from build123d import *

# Parameters (mm, degrees)
F1_DEPTH       = 25
F3_DEPTH       = 5
F2_R           = 2
F4_DEPTH       = 7.001
F6_D           = 4
F6_CBORE_D     = 7.5
F6_CBORE_DEPTH = 2.5
F7_R           = 10
F8_DEPTH       = 2
F9_R           = 2.5


with BuildPart() as f1:
    # F0 (on Right) → F1 (new body)
    with BuildSketch(Plane.YZ):
        with BuildLine():
            Line((24, 25), (-24, 25))
            ThreePointArc((-24, 25), (-32.4852813742, 21.4852813742), (-36, 13))
            Line((-36, 13), (-36, 10))
            ThreePointArc((-36, 10), (-34.6554428129, 4.480802734), (-30.9230769231, 0.1984181931))
            ThreePointArc((-30.9230769231, 0.1984181931), (-30.6120464323, -0.1584471853), (-30.5, -0.6183802908))
            Line((-30.5, -0.6183802908), (-30.5, -41.5))
            ThreePointArc((-30.5, -41.5), (-30.2071067812, -42.2071067812), (-29.5, -42.5))
            Line((-29.5, -42.5), (-28.9142135624, -42.5))
            ThreePointArc((-28.9142135624, -42.5), (-28.53153013, -42.4238795325), (-28.2071067812, -42.2071067812))
            Line((-28.2071067812, -42.2071067812), (-26.2928932188, -40.2928932188))
            ThreePointArc((-26.2928932188, -40.2928932188), (-26.0761204675, -39.96846987), (-26, -39.5857864376))
            Line((-26, -39.5857864376), (-26, -39))
            Line((-26, -39), (-27, -39))
            Line((-27, -39), (-27, -37))
            Line((-27, -37), (-26, -37))
            Line((-26, -37), (-26, -36.4142135624))
            ThreePointArc((-26, -36.4142135624), (-26.0761204675, -36.03153013), (-26.2928932188, -35.7071067812))
            Line((-26.2928932188, -35.7071067812), (-28.2071067812, -33.7928932188))
            ThreePointArc((-28.2071067812, -33.7928932188), (-28.4238795325, -33.46846987), (-28.5, -33.0857864376))
            Line((-28.5, -33.0857864376), (-28.5, -11.4142135624))
            ThreePointArc((-28.5, -11.4142135624), (-28.4238795325, -11.03153013), (-28.2071067812, -10.7071067812))
            Line((-28.2071067812, -10.7071067812), (-27.7928932188, -10.2928932188))
            ThreePointArc((-27.7928932188, -10.2928932188), (-27.5761204675, -9.96846987), (-27.5, -9.5857864376))
            Line((-27.5, -9.5857864376), (-27.5, -9))
            Line((-27.5, -9), (-28.5, -9))
            Line((-28.5, -9), (-28.5, -7))
            Line((-28.5, -7), (-27.5, -7))
            Line((-27.5, -7), (-27.5, -6.4142135624))
            ThreePointArc((-27.5, -6.4142135624), (-27.5761204675, -6.03153013), (-27.7928932188, -5.7071067812))
            Line((-27.7928932188, -5.7071067812), (-28.2071067812, -5.2928932188))
            ThreePointArc((-28.2071067812, -5.2928932188), (-28.4238795325, -4.96846987), (-28.5, -4.5857864376))
            Line((-28.5, -4.5857864376), (-28.5, -2.5199840255))
            ThreePointArc((-28.5, -2.5199840255), (-28.1044705248, -1.7233565187), (-27.2307692308, -1.5569083313))
            ThreePointArc((-27.2307692308, -1.5569083313), (-25.6305060602, -1.8887110314), (-24, -2))
            Line((-24, -2), (24, -2))
            ThreePointArc((24, -2), (25.6305060602, -1.8887110314), (27.2307692308, -1.5569083313))
            ThreePointArc((27.2307692308, -1.5569083313), (28.1044705248, -1.7233565187), (28.5, -2.5199840255))
            Line((28.5, -2.5199840255), (28.5, -4.5857864376))
            ThreePointArc((28.5, -4.5857864376), (28.4238795325, -4.96846987), (28.2071067812, -5.2928932188))
            Line((28.2071067812, -5.2928932188), (27.7928932188, -5.7071067812))
            ThreePointArc((27.7928932188, -5.7071067812), (27.5761204675, -6.03153013), (27.5, -6.4142135624))
            Line((27.5, -6.4142135624), (27.5, -7))
            Line((27.5, -7), (28.5, -7))
            Line((28.5, -7), (28.5, -9))
            Line((28.5, -9), (27.5, -9))
            Line((27.5, -9), (27.5, -9.5857864376))
            ThreePointArc((27.5, -9.5857864376), (27.5761204675, -9.96846987), (27.7928932188, -10.2928932188))
            Line((27.7928932188, -10.2928932188), (28.2071067812, -10.7071067812))
            ThreePointArc((28.2071067812, -10.7071067812), (28.4238795325, -11.03153013), (28.5, -11.4142135624))
            Line((28.5, -11.4142135624), (28.5, -33.0857864376))
            ThreePointArc((28.5, -33.0857864376), (28.4238795325, -33.46846987), (28.2071067812, -33.7928932188))
            Line((28.2071067812, -33.7928932188), (26.2928932188, -35.7071067812))
            ThreePointArc((26.2928932188, -35.7071067812), (26.0761204675, -36.03153013), (26, -36.4142135624))
            Line((26, -36.4142135624), (26, -37))
            Line((26, -37), (27, -37))
            Line((27, -37), (27, -39))
            Line((27, -39), (26, -39))
            Line((26, -39), (26, -39.5857864376))
            ThreePointArc((26, -39.5857864376), (26.0761204675, -39.96846987), (26.2928932188, -40.2928932188))
            Line((26.2928932188, -40.2928932188), (28.2071067812, -42.2071067812))
            ThreePointArc((28.2071067812, -42.2071067812), (28.53153013, -42.4238795325), (28.9142135624, -42.5))
            Line((28.9142135624, -42.5), (29.5, -42.5))
            ThreePointArc((29.5, -42.5), (30.2071067812, -42.2071067812), (30.5, -41.5))
            Line((30.5, -41.5), (30.5, -0.6183802908))
            ThreePointArc((30.5, -0.6183802908), (30.6120464323, -0.1584471853), (30.9230769231, 0.1984181931))
            ThreePointArc((30.9230769231, 0.1984181931), (34.6554428129, 4.480802734), (36, 10))
            Line((36, 10), (36, 13))
            ThreePointArc((36, 13), (32.4852813742, 21.4852813742), (24, 25))
        make_face()
        with BuildLine():
            Line((24, 0), (-24, 0))
            ThreePointArc((-24, 0), (-31.0710678119, 2.9289321881), (-34, 10))
            Line((-34, 10), (-34, 13))
            ThreePointArc((-34, 13), (-31.0710678119, 20.0710678119), (-24, 23))
            Line((-24, 23), (24, 23))
            ThreePointArc((24, 23), (31.0710678119, 20.0710678119), (34, 13))
            Line((34, 13), (34, 10))
            ThreePointArc((34, 10), (31.0710678119, 2.9289321881), (24, 0))
        make_face(mode=Mode.SUBTRACT)
    extrude(amount=F1_DEPTH)

    # F3 (add): a face of the model
    f3_faces = [f1.faces().sort_by_distance(p)[0] for p in [
        (12.5, 0, 25),
    ]]
    extrude(f3_faces, amount=F3_DEPTH)

    # F2 (on face) → F4 (cut, through all)
    with BuildSketch(Plane(origin=(0, 0, 23), x_dir=(1, 0, 0), z_dir=(0, 0, -1))):
        with Locations((7, 0)):
            Circle(F2_R)
        with Locations((12.5, -5.5)):
            Circle(F2_R)
        with Locations((18, 0)):
            Circle(F2_R)
        with Locations((12.5, 5.5)):
            Circle(F2_R)
    extrude(amount=-F4_DEPTH, mode=Mode.SUBTRACT)

    # F6 (through all)
    with Locations(Plane(origin=(0, 0, 23), x_dir=(1, 0, 0), z_dir=(0, 0, -1))):
        with Locations((12.5, -5.5), (7, 0), (18, 0), (12.5, 5.5)):
            CounterBoreHole(F6_D / 2, F6_CBORE_D / 2, F6_CBORE_DEPTH)

    # F7 (on face) → F8 (cut, through all)
    with BuildSketch(Plane(origin=(0, 0, -2), x_dir=(1, 0, 0), z_dir=(0, 0, -1))):
        with Locations((12.5, 0)):
            Circle(F7_R)
    extrude(amount=-F8_DEPTH, mode=Mode.SUBTRACT)

    # F9
    f9_edges = [f1.edges().sort_by_distance(p)[0] for p in [
        (12.5, -24, 25),
        (12.5, 24, 25),
        (12.5, 24, 30),
        (12.5, -24, 30),
    ]]
    fillet(f9_edges, radius=F9_R)


solid = f1.part
The model under review builds one solid part; all positions refer to its coordinate system, in mm. A direction names the side the tool comes from. Round coordinates to 2 decimals unless told otherwise and drop trailing zeros. Order: outer loops, then holes, each group sorted by start corner. A loop starts at its lowest first (then second) coordinate and runs counter-clockwise, first axis right, second up. Notation, with made-up numbers: (25, 84) -> (73, 84) arc R17 cw to (73, 100) -> close; hole circle Ø5 at (10, 51). An arc over 180 degrees is marked (long way). Return JSON: item names as keys, results as strings.
1. The part is to be moulded in two halves that separate along X. For faces 6 (the face through (12, -36, 12)), 7 (the face through (22.04, -3, -1.01)), say which applies: +X half, -X half, draft (parallel to the pull), parting line (faces both ways), or undercut.
Answer block:
{"face 6": "draft", "face 7": "undercut"}
2. Take a section at B-B (y = 0). Write out the cut boundary in (x, z), then the cut area to 4 significant figures.
Answer block:
{"outline": "(0, -2) -> (2.5, -2) -> (2.5, 0) -> (0, 0) -> close; (0, 23) -> (3.25, 23) -> (3.25, 25.5) -> (5, 25.5) -> (5, 30) -> (0, 30) -> close; (9, 25.5) -> (10.75, 25.5) -> (10.75, 23) -> (14.25, 23) -> (14.25, 25.5) -> (16, 25.5) -> (16, 30) -> (9, 30) -> close; (20, 25.5) -> (21.75, 25.5) -> (21.75, 23) -> (25, 23) -> (25, 30) -> (20, 30) -> close; (22.5, -2) -> (25, -2) -> (25, 0) -> (22.5, 0) -> close", "area": "111.5 mm²"}
3. Take a section at D-D (x = 12.5). State how many separate pieces and enclosed holes the cut face has, then the cut area to 3 significant figures.
Answer block:
{"separate pieces": "3", "enclosed holes": "0", "area": "670 mm²"}
4. For L1, parallel to X at y = 0, z = 28; L2, parallel to Y at x = 11.5, z = -16; L3, parallel to Z at x = 16, y = 17.5, list the stretches that pass through material, from the lowest coordinate up. Write a range as [from, to].
Answer block:
{"L1": "x = [0, 5], [9, 16], [20, 25]", "L2": "y = [-30.5, -28.5], [28.5, 30.5]", "L3": "z = [-2, 0], [23, 30]"}
5. Insertion check: P1, Ø12, axis at x = 10, z = -23, coming from the -Y side; P2, Ø3, axis at x = 7, y = 0, coming from the +Z side; P3, Ø0.8, axis at x = 14.5, y = 28, coming from the -Z side; P4, Ø12.5, axis at x = 10, y = 0.5, coming from the -Z side. Each pin has a flat end and moves straight along its axis. Give the tip position at first contact, or say it passes through.
Answer block:
{"P1": "stops at y = -30.5", "P2": "passes through", "P3": "stops at z = -42.36", "P4": "stops at z = 23"}
6. For faces 1 (the face through (12, -28.5, -8)), 2 (the face through (3.254, -0.165, 24.232)), 3 (the face through (10.9, 6.7, 27.7)), 4 (the face through (12.675, 24.57, 25.693)), 5 (the face through (12, 30.5, -21)), list the 3-axis set-ups (+Z, -Z, +X, -X, +Y, -Y) from which the entire face can be reached by the end or side of a thin tool; tool diameter is ignored.
Answer block:
{"face 1": "+X, -X", "face 2": "-Z", "face 3": "+Z, -Z", "face 4": "+Z, +X, -X, +Y", "face 5": "-Z, +X, -X, +Y"}
7. Take a section at C-C (z = -21). Write out the cut boundary in (x, y).
Answer block:
{"outline": "(0, -30.5) -> (25, -30.5) -> (25, -28.5) -> (0, -28.5) -> close; (0, 28.5) -> (25, 28.5) -> (25, 30.5) -> (0, 30.5) -> close"}
8. Take a section at A-A (y = 18). Write out the cut boundary in (x, z).
Answer block:
{"outline": "(0, -2) -> (25, -2) -> (25, 0) -> (0, 0) -> close; (0, 23) -> (25, 23) -> (25, 30) -> (0, 30) -> close"}
